Design review of the part built by this model. Coordinates are the model's own, in mm. Face numbers are marked on the shaded views. Round coordinates to 2 decimals unless told otherwise and drop trailing zeros. Order: outer loops, then holes, each group sorted by start corner. A loop starts at its lowest first (then second) coordinate and runs counter-clockwise, first axis right, second up.
Autodesk Inventor part; units mm, degrees
ref_plane "YZ Plane" through (0, 0, 0) normal (1, 0, 0) x (0, 1, 0)
ref_plane "XZ Plane" through (0, 0, 0) normal (0, 1, 0) x (-1, 0, 0)
ref_plane "XY Plane" through (0, 0, 0) normal (0, 0, 1) x (1, 0, 0)
sketch "Sketch1" plane through (0, 0, 0) normal (1, 0, 0) x (0, 1, 0)
  line L0 (0, 0) -> (50.8, 0)
  line L1 (0, 138.1125) -> (26.719, 138.1125)
  line L2 (0, 138.1125) -> (0, 169.8625)
  line L3 (0, 169.8625) -> (3.175, 169.8625)
  line L4 (3.175, 169.8625) -> (3.175, 141.2875)
  line L5 (22.9489, 141.2875) -> (60.325, 141.2875)
  line L6 (60.325, 141.2875) -> (60.325, 179.3875)
  line L7 (60.325, 179.3875) -> (63.5, 179.3875)
  line L8 (63.5, 179.3875) -> (63.5, 138.1125)
  line L9 (63.5, 138.1125) -> (35.6489, 138.1125)
  line L10 (29.2989, 139.7) -> (22.9489, 139.7)
  line L11 (22.9489, 139.7) -> (22.9489, 141.2875)
  line L12 (29.2989, 139.7) -> (35.6489, 139.7)
  line L13 (35.6489, 139.7) -> (35.6489, 138.1125)
  line L14 (29.2989, 164.2178) -> (29.2989, 141.2875)
  point P0 (62.1333, 179.3875)
  dimension "d0" = 50.8
  dimension "d1" = 138.1125
  dimension "d2" = 31.75
  dimension "d3" = 3.175
  dimension "d4" = 3.175
  dimension "d5" = 57.15
  dimension "d6" = 38.1
  dimension "d7" = 3.175
  dimension "d13" = 26.1239
  dimension "d14" = 1.5875
  dimension "d15" = 6.35
  dimension "d16" = 6.35
revolve "Revolution1" add sketch "Sketch1" angle 360 about axis through (0, 0, 0) along (0, 1, 0)
ref_plane "Work Plane1" through (0, 62.1333, 179.3875) normal (0, 0, 1) x (1, 0, 0)
sketch "Sketch2" plane through (0, 62.1333, 179.3875) normal (0, 0, 1) x (1, 0, 0)
  arc A0 (6.35, -32.8344) -> (-6.35, -32.8344) centre (0, -32.8344) ccw
  line L0 (169.8625, -58.9583) -> (-169.8625, -58.9583)
  line L1 (-6.35, -32.8344) -> (-6.35, -39.1844)
  line L2 (141.2875, -39.1844) -> (-141.2875, -39.1844)
  line L3 (6.35, -32.8344) -> (6.35, -39.1844)
  line L4 (-6.35, -39.1844) -> (6.35, -39.1844)
  point P0 (0, -62.1333)
  dimension "d9" = 12.7
  dimension "d10" = 26.1239
extrude "Extrusion1" cut sketch "Sketch2" against normal through all
sketch "Sketch3" plane through (0, 63.5, 0) normal (0, 1, 0) x (1, 0, 0)
  line L0 (0, 0) -> (-271.4312, -271.4312)
  line L1 (0, 0) -> (383.8617, 0) construction
  line L2 (-271.4312, -271.4312) -> (-271.4312, 238.0261)
  line L3 (-271.4312, 238.0261) -> (250.2845, 238.0261)
  line L4 (0, 0) -> (271.4312, -271.4312)
  line L5 (0, 0) -> (383.8617, 0) construction
  line L6 (271.4312, -271.4312) -> (250.2845, 238.0261)
  dimension "d17" = 135
  dimension "d18" = 45
extrude "Extrusion2" cut sketch "Sketch3" against normal through all
properties part number "Layer2_Top_Quarter"
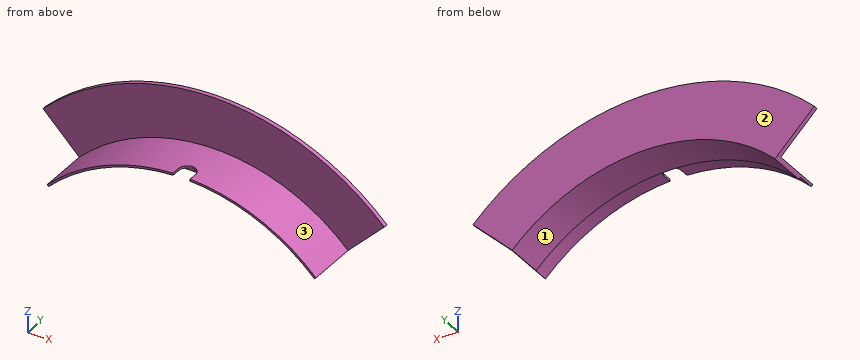
1) The part is to be moulded in two halves that separate along X. For the marked faces 1, 2 and 3, say which applies: released by +X, released by -X, zero draft, split by the parting line, or undercut.
Results:
face 1: undercut
face 2: zero draft
face 3: split by the parting line
2) Take a section at C-C on x = 77. Give the boundary of the cut face in (y, z) (3 decimals), plus the area to 3 significant figures.
Results:
outline: (22.949, 116.564) - (35.649, 116.564) - (35.649, 114.656) - (63.5, 114.656) - (63.5, 162.021) - (60.325, 162.021) - (60.325, 118.462) - (22.949, 118.462) - close
area: 268 mm2
3) Take a section at D-D on z = 103.5. Give the boundary of the cut face in (x, y) (3 decimals), plus the area to 3 significant figures.
Results:
outline: (-103.5, 60.325) - (-96.176, 60.325) - (-96.176, 22.949) - (-93.829, 22.949) - (-93.829, 35.649) - (-91.448, 35.649) - (-91.448, 63.5) - (-103.5, 63.5) - close; (91.448, 35.649) - (93.829, 35.649) - (93.829, 22.949) - (96.176, 22.949) - (96.176, 60.325) - (103.5, 60.325) - (103.5, 63.5) - (91.448, 63.5) - close
area: 369 mm2
4) Take a section at A-A on y = 32.5. Give the boundary of the cut face in (x, z) (1 decimal), plus the area to 3 significant figures.
Results:
outline: (-99.9, 99.9) - (-98.8, 98.8) arc R139.7 cw to (-5.5, 139.6) - (-5.5, 141.2) arc R141.3 ccw to start; (5.5, 139.6) arc R139.7 cw to (98.8, 98.8) - (99.9, 99.9) arc R141.3 ccw to (5.5, 141.2) - close
area: 333 mm2
5) Clearance check with flat-ended pins moving along their axes: P1, Ø2, axis at x = -71.5, y = 46.5, coming from the -Z side; P2, Ø1, axis at y = 31.5, z = 123.5, coming from the +X side; P3, Ø1.5, axis at x = 48.5, y = 42.5, coming from the +Z side. State where each tip first meets the part, or that it passes through.
Results:
P1: stops at z = 117.55
P2: stops at x = 69.52
P3: stops at z = 132.97
6) To check wall thickness, follow line 1 along Y through (x, z) = (-40.5, 146) (3 decimals); line 2 along X through (y, z) = (34, 104); line 3 along X through (y, z) = (46.5, 105). State the ranges of each line that lie inside material, in increasing order.
Results:
line 1: y = 60.325 to 63.5
line 2: x = -95.64 to -93.27, 93.27 to 95.64
line 3: x = -94.54 to -89.72, 89.72 to 94.54
7) Take a section at B-B on z = 123. Give the boundary of the cut face in (x, y) (3 decimals), plus the area to 3 significant figures.
Results:
outline: (-123, 60.325) - (-69.521, 60.325) - (-69.521, 22.949) - (-66.235, 22.949) - (-66.235, 35.649) - (-62.818, 35.649) - (-62.818, 63.5) - (-123, 63.5) - close; (62.818, 35.649) - (66.235, 35.649) - (66.235, 22.949) - (69.521, 22.949) - (69.521, 60.325) - (123, 60.325) - (123, 63.5) - (62.818, 63.5) - close
area: 796 mm2
